Autodesk Inventor part; units mm, degrees
ref_plane "YZ Plane" through (0, 0, 0) normal (1, 0, 0) x (0, 1, 0)
ref_plane "XZ Plane" through (0, 0, 0) normal (0, 1, 0) x (-1, 0, 0)
ref_plane "XY Plane" through (0, 0, 0) normal (0, 0, 1) x (1, 0, 0)
sketch "Эскиз1" plane through (0, 0, 0) normal (0, 0, 1) x (1, 0, 0)
  line L0 (2.2305, 14.4712) -> (2.2305, 9.7212)
  line L1 (2.2305, 9.7212) -> (-2.6195, 9.7212)
  line L2 (-2.6195, 9.7212) -> (-2.6195, 14.4712)
  line L3 (-2.6195, 14.4712) -> (2.2305, 14.4712)
  line L4 (7.3598, -20.4288) -> (7.3598, 19.5712)
  line L5 (7.3598, 19.5712) -> (2.8055, 19.5712)
  line L6 (2.8055, 19.5712) -> (2.8055, 24.5712)
  line L7 (2.8055, 24.5712) -> (-3.0445, 24.5712)
  line L8 (-3.0445, 24.5712) -> (-3.0445, 19.5712)
  line L9 (-3.0445, 19.5712) -> (-7.6402, 19.5712)
  line L10 (-7.6402, 19.5712) -> (-7.6402, -20.4288)
  line L11 (-7.6402, -20.4288) -> (-3.0445, -20.4288)
  line L12 (-3.0445, -20.4288) -> (-3.0445, -25.4288)
  line L13 (-3.0445, -25.4288) -> (2.8055, -25.4288)
  line L14 (2.8055, -25.4288) -> (2.8055, -20.4288)
  line L15 (2.8055, -20.4288) -> (7.3598, -20.4288)
  line L16 (2.2305, -10.4288) -> (2.2305, -15.1788)
  line L17 (2.2305, -15.1788) -> (-2.6195, -15.1788)
  line L18 (-2.6195, -15.1788) -> (-2.6195, -10.4288)
  line L19 (-2.6195, -10.4288) -> (2.2305, -10.4288)
extrude "Выдавливание1" add sketch "Эскиз1" along normal blind 4.9
properties part number "В. шарн. - соединитель"
CAD build for the part. Positions are in the model's coordinates, mm. A direction names the side the tool comes from. Round coordinates to 2 decimals unless told otherwise and drop trailing zeros. Write each loop counter-clockwise with the first axis right and the second up, starting at its lowest first coordinate (ties: lowest second). Pieces come first, ordered by that corner, then holes. Notation, with made-up numbers: (-24, 50.25) - (32, 50.25) arc R16 ccw to (32, 79.25) - close; hole circle Ø3 at (2.25, 39). An arc over 180 degrees is marked (long way). Return JSON: item names as keys, results as strings. Group by question number.
Item 1: Flat gauge pins, fed straight in: pin 1 Ø2.5 at (x, z) = (-6.5, 3.5) entering from +Y; pin 2 Ø1.5 at (y, z) = (22, 3) entering from +X; pin 3 Ø2.5 at (x, z) = (4.5, 1.5) entering from -Y. Where does each tip first touch, or does it go through?
Item 2: 3-axis set-ups, long thin cutter, end or side, ignore diameter. For faces 1 (the face through (-3.044, -23, 2)), 2 (the face through (5, -20.429, 2)), 3 (the face through (-3.044, 22, 2)), 4 (the face through (5, 19.571, 2)), 5 (the face through (0, 9.721, 2)): which of +Z, -Z, +X, -X, +Y, -Y reach the whole face in a straight line?
Item 3: Probe probe 1 along Y at (x, z) = (-0.25, 0.25); probe 2 along X at (y, z) = (-13.5, 2.5); probe 3 along Y at (x, z) = (5, 2.1). List the from-to ranges inside material, lowest first.
Item 4: Band-saw the part on A-A on x = -2. List the corners of the cut face in (y, z).
Item 5: Band-saw the part on B-B on z = 3.1. List the corners of the cut face in (x, y), plus the area to 3 significant figures.
Item 6: Band-saw the part on C-C on x = -4.75. List the corners of the cut face in (y, z).
Item 7: Mould opens along Y. For faces 6 (the face through (0, -15.179, 2)), 7 (the face through (0, -25.429, 2)), 8 (the face through (0, 0, 0)), 9 (the face through (-5, 19.571, 2)) say: +Y half, -Y half, draft (parallel to the pull), parting line (faces both ways), or undercut.
Resolved:
{
 "1": {"pin 1": "stops at y = 19.57", "pin 2": "stops at x = 2.81", "pin 3": "stops at y = -20.43"},
 "2": {"face 1": "+Z, -Z, -X, -Y", "face 2": "+Z, -Z, +X, -Y", "face 3": "+Z, -Z, -X, +Y", "face 4": "+Z, -Z, +X, +Y", "face 5": "+Z, -Z"},
 "3": {"probe 1": "y = -25.43 to -15.18, -10.43 to 9.72, 14.47 to 24.57", "probe 2": "x = -7.64 to -2.62, 2.23 to 7.36", "probe 3": "y = -20.43 to 19.57"},
 "4": {"outline": "(-25.43, 0) - (-15.18, 0) - (-15.18, 4.9) - (-25.43, 4.9) - close; (-10.43, 0) - (9.72, 0) - (9.72, 4.9) - (-10.43, 4.9) - close; (14.47, 0) - (24.57, 0) - (24.57, 4.9) - (14.47, 4.9) - close"},
 "5": {"outline": "(-7.64, -20.43) - (-3.04, -20.43) - (-3.04, -25.43) - (2.81, -25.43) - (2.81, -20.43) - (7.36, -20.43) - (7.36, 19.57) - (2.81, 19.57) - (2.81, 24.57) - (-3.04, 24.57) - (-3.04, 19.57) - (-7.64, 19.57) - close; hole (-2.62, -15.18) - (2.23, -15.18) - (2.23, -10.43) - (-2.62, -10.43) - close; hole (-2.62, 9.72) - (2.23, 9.72) - (2.23, 14.47) - (-2.62, 14.47) - close", "area": "612 mm²"},
 "6": {"outline": "(-20.43, 0) - (19.57, 0) - (19.57, 4.9) - (-20.43, 4.9) - close"},
 "7": {"face 6": "undercut", "face 7": "-Y half", "face 8": "draft", "face 9": "+Y half"}
}
